Solid Edge part; units mm, degrees
sketch "Sketch1" plane through (0, 0, 0) normal (0, 0, 1) x (1, 0, 0)
  line L0 (0, 0) -> (0, 8.25)
  line L1 (0, 8.25) -> (0.5, 8.25)
  line L2 (0.5, 8.25) -> (0.5, 8.3865)
  line L3 (0.5, 8.3865) -> (1.1135, 9)
  line L4 (1.1135, 9) -> (29.3865, 9)
  line L5 (29.3865, 9) -> (30, 8.3865)
  line L6 (30, 8.3865) -> (30, 4.5)
  arc A0 (30, 4.5) -> (31, 3.5) centre (31, 4.5) ccw
  line L7 (31, 3.5) -> (35, 3.5)
  line L8 (35, 3.5) -> (35, 3.3865)
  line L9 (35, 3.3865) -> (38.5, 3.3865)
  line L10 (38.5, 3.3865) -> (39.1135, 4)
  line L11 (39.1135, 4) -> (40.8865, 4)
  line L12 (40.8865, 4) -> (41.5, 3.3865)
  line L13 (41.5, 3.3865) -> (41.9657, 3.3865)
  line L14 (41.9657, 3.3865) -> (42.05, 3.45)
  line L15 (42.05, 3.45) -> (42.25, 3.45)
  line L16 (42.25, 3.45) -> (44, 3.25)
  line L17 (44, 3.25) -> (44, 0)
  line L18 (44, 0) -> (0, 0)
revolve "RevolvedProtrusion1" add sketch "Sketch1" angle 360 about axis through (44, 0, 0) along (-1, 0, 0)
cosmetic_thread "Thread1"
hole "Bohrung_1" at (44, 0, 0) direction (-1, 0, 0) diameter 5.8 depth 5
hole "Bohrung_2" at (36.9, 1.8738, 1.8738) direction (0, 0.7071, 0.7071) diameter 2 depth 0.75
hole "Bohrung_3" at (36.9, -1.8738, 1.8738) direction (0, -0.7071, 0.7071) diameter 2 depth 0.75
hole "Bohrung_4" at (36.9, -1.8738, -1.8738) direction (0, -0.7071, -0.7071) diameter 2 depth 0.75
hole "Bohrung_5" at (36.9, 1.8738, -1.8738) direction (0, 0.7071, -0.7071) diameter 2 depth 0.75
sketch "Sketch2" plane through (0, 0, 0) normal (0, 0, 1) x (1, 0, 0)
  line L0 (39, 1.75) -> (39, 2.25)
  line L1 (39, 2.25) -> (42.767, 2.25)
  line L2 (42.767, 2.25) -> (43.7, 2)
  line L3 (43.7, 2) -> (43.7, 1.75)
  line L4 (43.7, 1.75) -> (39, 1.75)
revolve "RevolvedProtrusion2" add sketch "Sketch2" angle 360 about axis through (43.7, 1.75, 0) along (-1, 0, 0)
sketch "Sketch3" plane through (0, 0, 0) normal (0, 0, 1) x (1, 0, 0)
  line L0 (39, -1.75) -> (39, -1.25)
  line L1 (39, -1.25) -> (42.767, -1.25)
  line L2 (42.767, -1.25) -> (43.7, -1.5)
  line L3 (43.7, -1.5) -> (43.7, -1.75)
  line L4 (43.7, -1.75) -> (39, -1.75)
revolve "RevolvedProtrusion3" add sketch "Sketch3" angle 360 about axis through (43.7, -1.75, 0) along (-1, 0, 0)
sketch "Sketch4" plane through (0, 0, -1.75) normal (0, 0, 1) x (1, 0, 0)
  line L0 (39, 0) -> (39, 0.5)
  line L1 (39, 0.5) -> (42.767, 0.5)
  line L2 (42.767, 0.5) -> (43.7, 0.25)
  line L3 (43.7, 0.25) -> (43.7, 0)
  line L4 (43.7, 0) -> (39, 0)
revolve "RevolvedProtrusion4" add sketch "Sketch4" angle 360 about axis through (43.7, 0, -1.75) along (-1, 0, 0)
properties part number "BALLUFF BES 516-326-G-E5-Y-S49_1"
The listing builds one solid part. Answer for the finished solid, in the listing's coordinates (mm). A direction names the side the tool comes from. Round coordinates to 2 decimals unless told otherwise and drop trailing zeros. Write each loop counter-clockwise with the first axis right and the second up, starting at its lowest first coordinate (ties: lowest second). Pieces come first, ordered by that corner, then holes. Notation, with made-up numbers: M 62,74.25 L 104,74.25 A32 ccw 104,109.25 Z; hole C 26.5,27 d10. An arc over 180 degrees is marked long. Write each question's results on one line, items separated by ' | '. Start each with the question number.
(1) Find the intervals of material crossed by line 1 (Y direction, x = 41.95, z = 0); line 2 (Y direction, x = 40.4, z = 0); line 3 (Z direction, x = 42.2, y = 0), in increasing order.
(2) Each of these flat-tipped pins is pushed along its axis until it touches: P1, Ø1, axis at x = 15, y = 2, coming from the -Z side; P2, Ø5, axis at x = 14, z = -6, coming from the +Y side; P3, Ø0.6, axis at y = 2, z = 0, coming from the +X side. Where does it stop, or does it pass through?
(3) The part is cut by section A-A, the plane x = 25.5. Write down the section's boundary in (y, z).
(4) For faces 1 (the cylindrical face through (0.25, 7.62, -3.16)), 2 (the cylindrical face through (40.91, 1.25, 0.02)), 3 (the flat face through (36.886, -1.864, -1.884)), determine the directions among +Z, -Z, +X, -X, +Y, -Y from which every point of the face is accessible in a straight line to the end or side of a thin tool.
(5) Determine the mould class of faces 4 (the conical face through (43.331, -2.007, -0.236)), 5 (the flat face through (36.886, 1.884, 1.864)), 6 (the flat face through (0, 0, 0)) for opening direction X: +X half, -X half, draft (parallel to the pull), parting line (faces both ways), or undercut.
Worked answers:
1) line 1: y = -3.39 to -2.9, -2.25 to -1.25, 1.25 to 2.25, 2.9 to 3.39 | line 2: y = -4 to -2.9, -2.25 to -1.25, 1.25 to 2.25, 2.9 to 4 | line 3: z = -3.45 to -2.9, -2.25 to -1.25, 2.9 to 3.45
2) P1: stops at z = -8.87 | P2: stops at y = 8.29 | P3: stops at x = 43.7
3) outline: C 0,0 d18
4) face 1: -X | face 2: +X | face 3: none
5) face 4: +X half | face 5: undercut | face 6: -X half
